Input: dimensioned drawing with shaded views. Units: mm. Origin: part minimum x, y, z. A direction names the side the tool comes from. Give positions to 0.01 mm unless a question says otherwise; leave off trailing zeros. Loops run counter-clockwise (first coordinate to the right, second up) from the corner with the lowest first, then second, coordinate; pieces in that order, holes last.
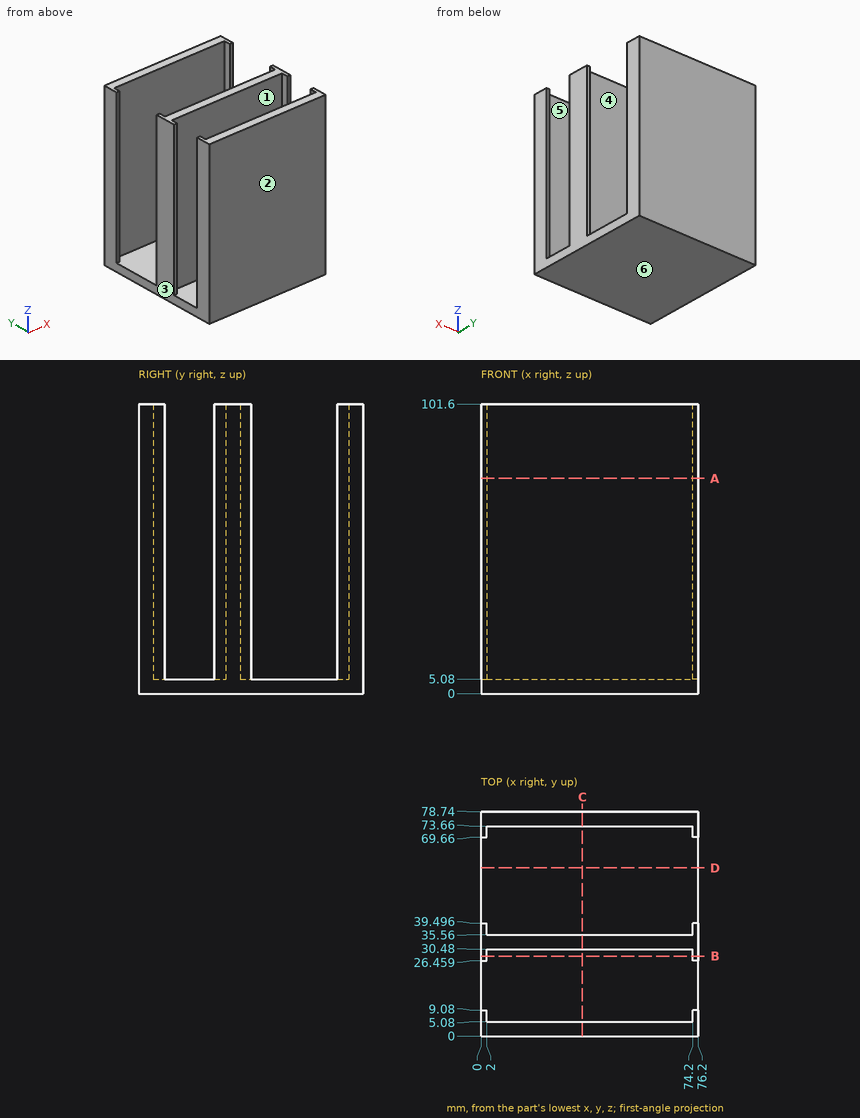
(1) Ray query, line 1 along Y through (x, z) = (64.5, 52.5); line 2 along X through (y, z) = (8.5, 83); line 3 along Z through (x, y) = (61, 11). Return the intervals inside material, ascending.
A:
line 1: y = 0 to 5.08, 30.48 to 35.56, 73.66 to 78.74
line 2: x = 0 to 2, 74.2 to 76.2
line 3: z = 0 to 5.08
(2) Section A-A, the plane z = 75.5. Return the cut outline in (x, y) (1 decimal).
A:
outline: (0, 0) - (76.2, 0) - (76.2, 9.1) - (74.2, 9.1) - (74.2, 5.1) - (2, 5.1) - (2, 9.1) - (0, 9.1) - close; (0, 26.5) - (2, 26.5) - (2, 30.5) - (74.2, 30.5) - (74.2, 26.5) - (76.2, 26.5) - (76.2, 39.5) - (74.2, 39.5) - (74.2, 35.6) - (2, 35.6) - (2, 39.5) - (0, 39.5) - close; (0, 69.7) - (2, 69.7) - (2, 73.7) - (74.2, 73.7) - (74.2, 69.7) - (76.2, 69.7) - (76.2, 78.7) - (0, 78.7) - close
(3) Section C-C, the plane x = 35.5. Return the cut outline in (y, z), then the cut area to 3 significant figures.
A:
outline: (0, 0) - (78.74, 0) - (78.74, 101.6) - (73.66, 101.6) - (73.66, 5.08) - (35.56, 5.08) - (35.56, 101.6) - (30.48, 101.6) - (30.48, 5.08) - (5.08, 5.08) - (5.08, 101.6) - (0, 101.6) - close
area: 1,870 mm2
(4) Section D-D, the plane y = 59. Return the cut outline in (x, z), then the cut area to 3 significant figures.
A:
outline: (0, 0) - (76.2, 0) - (76.2, 5.08) - (0, 5.08) - close
area: 387 mm2
(5) Reachability of the marked faces 5 and 6 from +Z, -Z, +X, -X, +Y, -Y: full face, straight path, thin tool, end or side. Return the list, or none.
A:
face 5: +Z
face 6: -Z, +X, -X, +Y, -Y
(6) Mould query, pull axis Y, two halves, no side actions, for the marked faces 1, 2, 3 and 4. Classes: pulls with the +Y half, pulls with the -Y half, needs draft (parallel to the pull), parting line crosses it, or undercut.
A:
face 1: undercut
face 2: pulls with the -Y half
face 3: needs draft
face 4: undercut
(7) First-contact query: pin 1 (4 mm diameter, centred on x = 67, y = 10.5, fed in from +Z). Flat tip, straight axial feed; report the tip coordinate or a pass-through.
A:
pin 1: stops at z = 5.08
(8) Section B-B, the plane y = 28. Return the cut outline in (x, z).
A:
outline: (0, 0) - (76.2, 0) - (76.2, 101.6) - (74.2, 101.6) - (74.2, 5.08) - (2, 5.08) - (2, 101.6) - (0, 101.6) - close
